For this review, take the finished solid that the model builds, in its own axes (mm). Coordinates: 2 decimals unless noted, no trailing zeros. Write each loop counter-clockwise with the first axis right and the second up, starting at its lowest first coordinate (ties: lowest second). Pieces come first, ordered by that corner, then holes.
1) We need section A-A on z = -0.45. Write out the cut boundary in (x, y).
2) We need section D-D on x = 6.5. Write out the cut boundary in (y, z), then the cut area to 3 significant figures.
3) We need section C-C on y = 0. Write out the cut boundary in (x, z).
4) To check wall thickness, follow line 1 along Y through (x, z) = (0, -2.25); line 2 along Y through (x, z) = (1, -2.55); line 3 along X through (y, z) = (21, -2.7). State the ranges of each line that lie inside material, in increasing order.
5) Insertion check: P1, Ø0.9, axis at y = 68.5, z = -2, coming from the +X side. The pin has a flat end and moves straight along its axis. Give the tip position at first contact, or say it passes through.
6) We need section B-B on x = -1. Write out the cut boundary in (y, z), then the cut area to 3 significant figures.
from build123d import *

# Parameters (mm, degrees)
BOSS_EXTRUDE1_DEPTH = 3
SKETCH2_R           = 2.3
CUT_EXTRUDE1_DEPTH  = 10
SKETCH4_W           = 3
SKETCH4_H           = 20
BOSS_EXTRUDE3_DEPTH = 3


with BuildPart() as part:
    # Sketch1 → Boss-Extrude1 (new body)
    with BuildSketch(Plane.XY):
        with BuildLine():
            Line((-16.33027103, 11.546525368), (25, 70))
            Line((25, 70), (25, 40))
            Line((25, 40), (19.854388756, -2.408992972))
            ThreePointArc((19.854388756, -2.408992972), (-7.196803073, -18.660279353), (-16.33027103, 11.546525368))
        make_face()
    extrude(amount=-BOSS_EXTRUDE1_DEPTH)

    # Sketch2 → Cut-Extrude1 (cut)
    with BuildSketch(Plane.XY):
        Circle(SKETCH2_R)
    extrude(amount=-CUT_EXTRUDE1_DEPTH, mode=Mode.SUBTRACT)

    # Sketch4 → Boss-Extrude3 (add)
    with BuildSketch(Plane(origin=(25, 0, 0), x_dir=(0, 0, -1), z_dir=(1, 0, 0))):
        with Locations((1.5, 55)):
            Rectangle(SKETCH4_W, SKETCH4_H)
    extrude(amount=BOSS_EXTRUDE3_DEPTH)


solid = part.part
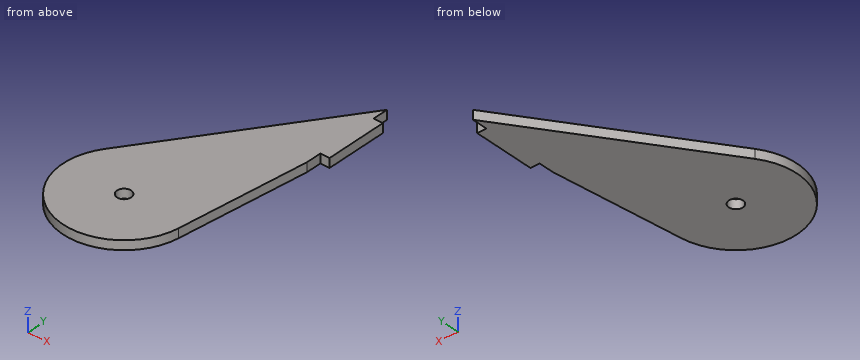
Result:
1. outline: (-16.33, 11.55) arc R20 ccw (long way) to (19.85, -2.41) - (25, 40) - (25, 45) - (28, 45) - (28, 65) - (25, 65) - (25, 70) - close; hole circle Ø4.6 at (0, 0)
2. outline: (-18.91, -3) - (43.84, -3) - (43.84, 0) - (-18.91, 0) - close
2. area: 188 mm2
3. outline: (-20, -3) - (-2.3, -3) - (-2.3, 0) - (-20, 0) - close; (2.3, -3) - (20.15, -3) - (20.15, 0) - (2.3, 0) - close
4. line 1: y = -20 to -2.3, 2.3 to 34.64
4. line 2: y = -19.97 to -2.07, 2.07 to 36.06
4. line 3: x = -9.65 to 22.69
5. P1: stops at x = 25
6. outline: (-19.97, -3) - (-2.07, -3) - (-2.07, 0) - (-19.97, 0) - close; (2.07, -3) - (33.23, -3) - (33.23, 0) - (2.07, 0) - close
6. area: 147 mm2
